Input: dimensioned drawing with shaded views. Units: mm. Origin: part minimum x, y, z. A direction names the side the tool comes from. Coordinates: 2 decimals unless noted, no trailing zeros. Loops run counter-clockwise (first coordinate to the right, second up) from the corner with the lowest first, then second, coordinate; pieces in that order, holes last.
(1) Section B-B, the plane z = 1.1. Return loops of the section in (x, y) (3 decimals), then the cut area to 3 significant figures.
(2) Section C-C, the plane x = 36. Return loops of the section in (y, z), then the cut area to 4 significant figures.
(3) Line query: L1, parallel to Y at x = 38.5, z = 1.8; L2, parallel to Y at x = 19.5, z = 2.4; L3, parallel to X at y = 6.25, z = 2.85. Output: solid intervals per line, ascending.
(4) Contact query for flat-ended pins moving along their axis: P1, Ø1.5, axis at y = 21.5, z = 2, coming from the +X side (3 decimals); P2, Ø1.5, axis at y = 22.5, z = 1, coming from the -X side (3 decimals); P3, Ø1.5, axis at x = 3.5, z = 2, coming from the +Y side. Output: stop coordinate, or through.
(5) Set-up query: the marked faces 3, 4, 5 and 6. Return all of +Z, -Z, +X, -X, +Y, -Y with unobstructed straight access to the full face (end or side cutting, diameter ignored); none if empty.
(6) Section D-D, the plane y = 3.5. Return loops of the section in (x, z), then the cut area to 3 significant figures.
(7) Section A-A, the plane y = 7.5. Return loops of the section in (x, z).
(8) Mould query, pull axis X, two halves, no side actions, for the marked faces 1 and 2. Classes: released by +X, released by -X, zero draft, split by the parting line, or undercut.
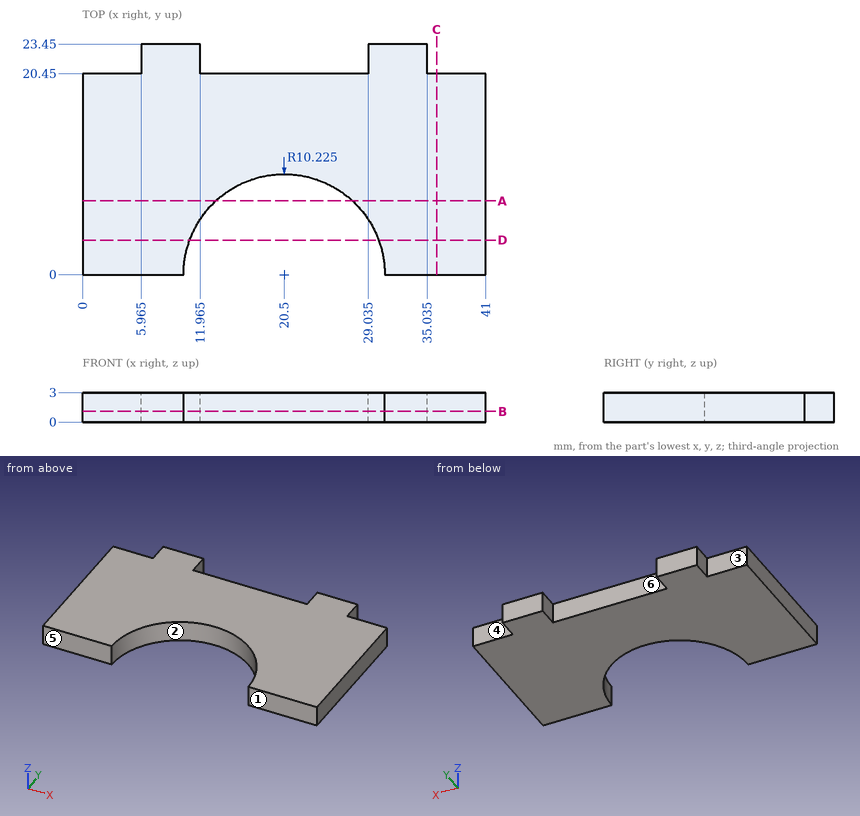
Report:
1. outline: (0, 0) - (10.275, 0) arc R10.225 cw to (30.725, 0) - (41, 0) - (41, 20.45) - (35.035, 20.45) - (35.035, 23.45) - (29.035, 23.45) - (29.035, 20.45) - (11.965, 20.45) - (11.965, 23.45) - (5.965, 23.45) - (5.965, 20.45) - (0, 20.45) - close
1. area: 710 mm2
2. outline: (0, 0) - (20.45, 0) - (20.45, 3) - (0, 3) - close
2. area: 61.35 mm2
3. L1: y = 0 to 20.45
3. L2: y = 10.18 to 20.45
3. L3: x = 0 to 12.41, 28.59 to 41
4. P1: stops at x = 35.035
4. P2: stops at x = 5.965
4. P3: stops at y = 20.45
5. face 3: +Z, -Z, -X, +Y
5. face 4: +Z, -Z, +X, +Y
5. face 5: +Z, -Z, +X, -X, -Y
5. face 6: +Z, -Z, +Y
6. outline: (0, 0) - (10.89, 0) - (10.89, 3) - (0, 3) - close; (30.11, 0) - (41, 0) - (41, 3) - (30.11, 3) - close
6. area: 65.4 mm2
7. outline: (0, 0) - (13.55, 0) - (13.55, 3) - (0, 3) - close; (27.45, 0) - (41, 0) - (41, 3) - (27.45, 3) - close
8. face 1: zero draft
8. face 2: undercut
